from build123d import *

# Parameters (mm, degrees)
SKETCH_W         = 17
SKETCH_H         = 22
PAD_DEPTH        = 2
SKETCH001_W      = 4
SKETCH001_H      = 22
PAD001_DEPTH     = 31
SKETCH002_R      = 10.75
SKETCH003_R      = 9.5
FILLET_R         = 2
HOLE_D           = 6
HOLE_DEPTH       = 26.197418
HOLE_CSINK_D     = 11.2
HOLE_CSINK_ANGLE = 90
HOLE_TIPS_R      = 3
FILLET001_R      = 5


with BuildPart() as part:
    # Sketch → Pad (new body)
    with BuildSketch(Plane.XY):
        with Locations((8.5, 11)):
            Rectangle(SKETCH_W, SKETCH_H)
    extrude(amount=PAD_DEPTH)

    # Sketch001 (on Face6 of Pad) → Pad001 (join)
    with BuildSketch(Plane.XY.offset(2)):
        with Locations((15, 11)):
            Rectangle(SKETCH001_W, SKETCH001_H)
        with Locations((2, 11)):
            Rectangle(SKETCH001_W, SKETCH001_H)
    extrude(amount=PAD001_DEPTH)

    # Sketch002 (on Face9 of Pad001) → AdditiveLoft section 0
    with BuildSketch(Plane(origin=(0, 0, 0), x_dir=(0, -1, 0), z_dir=(-1, 0, 0))):
        with Locations((-11, 22)):
            Circle(SKETCH002_R)
    # Sketch003 (on Face9 of Pad001) → AdditiveLoft section 1
    with BuildSketch(Plane(origin=(-26, 0, 0), x_dir=(0, -1, 0), z_dir=(-1, 0, 0))):
        with Locations((-11, 22)):
            Circle(SKETCH003_R)
    loft()

    # Fillet
    fillet_edges = [part.edges().sort_by_distance(p)[0] for p in [
        (-26, 20.5, 22),
    ]]
    fillet(fillet_edges, radius=FILLET_R)

    # Hole
    with Locations(Plane.YZ.offset(17)):
        with Locations((11, 22)):
            CounterSinkHole(HOLE_D / 2, HOLE_CSINK_D / 2, depth=HOLE_DEPTH, counter_sink_angle=HOLE_CSINK_ANGLE)

    # Hole tips → Hole tip 1 section 0
    with BuildSketch(Plane.YZ.offset(-9.197418), mode=Mode.PRIVATE) as hole_tip_1_s0:
        with Locations((11, 22)):
            Circle(HOLE_TIPS_R)
    loft([hole_tip_1_s0.sketch, Vertex(-11, 11, 22)], mode=Mode.SUBTRACT)

    # Fillet001
    fillet001_edges = [part.edges().sort_by_distance(p)[0] for p in [
        (15, 0, 33),
        (2, 0, 33),
        (2, 22, 33),
        (15, 22, 33),
    ]]
    fillet(fillet001_edges, radius=FILLET001_R)


solid = part.part
Source: CAD feature listing. Evaluate the final solid. Frame: model axes, mm. A direction names the side the tool comes from. Coordinates: 2 decimals unless noted, no trailing zeros. Loops run counter-clockwise (first coordinate to the right, second up) from the corner with the lowest first, then second, coordinate; pieces in that order, holes last. Notation, with made-up numbers: (12, 48.25) - (70, 48.25) arc R15 cw to (70, 63.25) - close; hole circle Ø1 at (69, 79.25). An arc over 180 degrees is marked (long way). Return JSON: item names as keys, results as strings.
Q1. Mould query, pull axis X, two halves, no side actions, for faces 5 (the flat face through (17, 11, 16)), 6 (the flat face through (4, 11, 17)), 7 (the flat face through (3, 22, 14)). Classes: released by +X, released by -X, zero draft, split by the parting line, or undercut.
Results:
{"face 5": "released by +X", "face 6": "undercut", "face 7": "zero draft"}
Q2. Contact query for flat-ended pins moving along their axis: P1, Ø1.5, axis at x = -1, y = 7, coming from the -Z side; P2, Ø11, axis at y = 16, z = 16, coming from the -X side; P3, Ø5, axis at y = 11, z = 22, coming from the +X side; P4, Ø1.5, axis at x = -9.5, y = 4, coming from the +Z side. Output: stop coordinate, or through.
Results:
{"P1": "z = 11.8", "P2": "x = -26", "P3": "x = -9.5", "P4": "z = 30.18"}
Q3. Section A-A, the plane x = 3. Return loops of the section in (y, z).
Results:
{"outline": "(0, 0) - (22, 0) - (22, 28) arc R5 ccw to (17, 33) - (5, 33) arc R5 ccw to (0, 28) - close; hole circle Ø6 at (11, 22)"}
Q4. Material intervals for line 1 along Z through (x, y) = (13.5, 11); line 2 along X through (y, z) = (16.5, 18.5); line 3 along X through (y, z) = (4.5, 5.5), sorted ascending.
Results:
{"line 1": "0 to 19, 25 to 33", "line 2": "-26 to 4, 13 to 17", "line 3": "0 to 4, 13 to 17"}
Q5. Access query for faces 1 (the cylindrical face through (-2.7, 13.4, 20.2)), 2 (the flat face through (8, 11, 2)), 3 (the flat face through (0, 11, 9)), 4 (the cylindrical face through (15, 1, 31)). Directions: +Z, -Z, +X, -X, +Y, -Y. A direction counts if a zero-diameter tool reaches every point of the face in a straight line with its end or side. Return the directions, or none.
Results:
{"face 1": "+X", "face 2": "+Z, +Y, -Y", "face 3": "-X", "face 4": "+Z, +X, -X, -Y"}
